The listing builds one solid part. Answer for the finished solid, in the listing's coordinates (mm). Face numbers are marked on the shaded views. A direction names the side the tool comes from. Round coordinates to 2 decimals unless told otherwise and drop trailing zeros. Write each loop counter-clockwise with the first axis right and the second up, starting at its lowest first coordinate (ties: lowest second). Pieces come first, ordered by that corner, then holes.
Item 1: Each of these flat-tipped pins is pushed along its axis until it touches: pin 1 (2 mm diameter, centred on x = -5, y = 16.5, fed in from -Z); pin 2 (0.8 mm diameter, centred on y = 13, z = 1, fed in from -X); pin 3 (2 mm diameter, centred on y = 21, z = 0, fed in from +X) (3 decimals); pin 4 (3.5 mm diameter, centred on x = 0, y = 44, fed in from +Z). Where does it stop, or does it pass through?
Item 2: Find section A-A on y = 16. Give the vertices of the cut face in (x, z) (3 decimals), then the cut area to 4 significant figures.
Item 3: For a pull along Y with two mould halves and no side action, classify the marked faces 1, 2, 3 and 4 as +Y half, -Y half, draft (parallel to the pull), parting line (faces both ways), or undercut.
Item 4: Find section B-B on y = 25. Give the vertices of the cut face in (x, z).
Item 5: Find the intervals of material crossed by probe 1 along X at (y, z) = (36, 0.75); probe 2 along X at (y, z) = (20, -1.25) (3 decimals); probe 3 along Z at (x, y) = (1, 45), in increasing order.
Item 6: A tool of negligible diameter and unlimited length cuts with its end or side. For the marked faces 5, 6 and 7, from which of +Z, -Z, +X, -X, +Y, -Y can it reach the whole face along a straight path? Write none if from no direction.
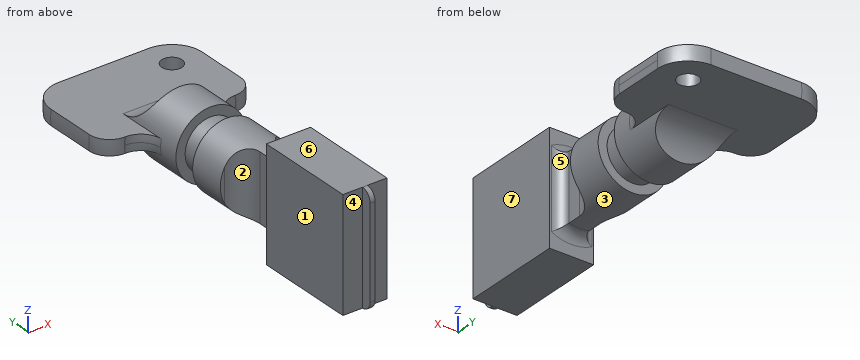
```python
from build123d import *

# Parameters (mm, degrees)
BOSS_EXTRUDE1_DEPTH      = 10
FILLET2_R                = 2
FILLET3_R                = 3
CUT_EXTRUDE1_DEPTH       = 49.473897211
CUT_EXTRUDE1_DEPTH_BACK  = 49.473897211
SKETCH3_R                = 1
CUT_EXTRUDE2_DEPTH       = 49.473897211
CUT_EXTRUDE2_DEPTH_BACK  = 49.473897211
SKETCH4_W                = 5.555619824
SKETCH4_H                = 11.886700215
SKETCH4_W_2              = 4.837610552
SKETCH4_H_2              = 13.886700215
FILLET4_R                = 2
BOSS_EXTRUDE2_DEPTH      = 5.5
BOSS_EXTRUDE2_DEPTH_BACK = 5.5
SKETCH7_W                = 4.35
SKETCH7_H                = 10
FILLET5_R                = 1
SKETCH8_W                = 0.486068648
SKETCH8_H                = 11
BOSS_EXTRUDE3_DEPTH      = 1
FILLET6_R                = 1


with BuildPart() as part:
    # Sketch1 → Revolve1 (revolve)
    with BuildSketch(Plane.XY):
        Polygon((-3.448914015, 37.765821371), (-3.448914015, 33.765821371), (-2.534753992, 33.765821371), (-2.534753992, 31.624967984), (-3.41766068, 31.624967984), (-3.41766068, 23), (0, 23), (0, 37.765821371), align=None)
    revolve(axis=Axis((0, 37.765821371, 0), (0, -1, 0)))

    # Sketch2 → Boss-Extrude1 (add)
    with BuildSketch(Plane(origin=(0, 37.765821371, 0), x_dir=(1, 0, 0), z_dir=(0, 1, 0))):
        with BuildLine():
            Line((3.366379046, 0.75), (-3.366379046, 0.75))
            ThreePointArc((-3.366379046, 0.75), (-3.448914015, 0), (-3.366379046, -0.75))
            Line((-3.366379046, -0.75), (3.366379046, -0.75))
            ThreePointArc((3.366379046, -0.75), (3.428218178, -0.37726384), (3.448914015, 0))
            ThreePointArc((3.448914015, 0), (3.428218178, 0.37726384), (3.366379046, 0.75))
        make_face()
        with BuildLine():
            Line((-3.366379046, 0.75), (-7.462405778, 0.75))
            ThreePointArc((-7.462405778, 0.75), (-7.5, 0), (-7.462405778, -0.75))
            Line((-7.462405778, -0.75), (-3.366379046, -0.75))
            ThreePointArc((-3.366379046, -0.75), (-3.448914015, 0), (-3.366379046, 0.75))
        make_face()
        with BuildLine():
            ThreePointArc((7.5, 0), (7.490595548, 0.375470813), (7.462405778, 0.75))
            Line((7.462405778, 0.75), (3.366379046, 0.75))
            ThreePointArc((3.366379046, 0.75), (3.428218178, 0.37726384), (3.448914015, 0))
            ThreePointArc((3.448914015, 0), (3.428218178, -0.37726384), (3.366379046, -0.75))
            Line((3.366379046, -0.75), (7.462405778, -0.75))
            ThreePointArc((7.462405778, -0.75), (7.490595548, -0.375470813), (7.5, 0))
        make_face()
    extrude(amount=BOSS_EXTRUDE1_DEPTH)

    # Fillet2
    # the kernel refuses this fillet: 2 mm, written as the material it adds along each edge
    with BuildSketch(Plane(origin=(0, 37.765821371, 0), x_dir=(-0.09803421101524086, 0, -0.9951830452085783), z_dir=(-0.9951830452085783, 0, 0.09803421101524086))) as fillet2_piece_1_section:
        with BuildLine():
            CenterArc((3.448914015 + FILLET2_R, FILLET2_R), FILLET2_R, 180, 90)
            Line((3.448914015 + FILLET2_R, 0), (3.448914015, 0))
            Line((3.448914015, 0), (3.448914015, FILLET2_R))
        make_face()
    fillet2_piece_1 = revolve(axis=Axis((0, 37.765821371, 0), (0, -1, 0)), revolution_arc=191.251965623, mode=Mode.PRIVATE)
    fillet2_piece_1 = split(fillet2_piece_1, bisect_by=Plane(origin=(3.870689991, 37.318827735, -0.75), z_dir=(0, 0, 1)), keep=Keep.TOP, mode=Mode.PRIVATE)
    fillet2_piece_1 = split(fillet2_piece_1, bisect_by=Plane(origin=(3.870689991, 37.318827735, 0.75), z_dir=(0, 0, -1)), keep=Keep.TOP, mode=Mode.PRIVATE)
    add(fillet2_piece_1)
    with BuildSketch(Plane(origin=(0, 37.765821371, 0), x_dir=(0.09800035789508027, 0, 0.9951863794548418), z_dir=(0.9951863794548418, 0, -0.09800035789508027))) as fillet2_piece_2_section:
        with BuildLine():
            CenterArc((3.448914015 + FILLET2_R, FILLET2_R), FILLET2_R, 180, 90)
            Line((3.448914015 + FILLET2_R, 0), (3.448914015, 0))
            Line((3.448914015, 0), (3.448914015, FILLET2_R))
        make_face()
    fillet2_piece_2 = revolve(axis=Axis((0, 37.765821371, 0), (0, -1, 0)), revolution_arc=95.624033786, mode=Mode.PRIVATE)
    fillet2_piece_2 = split(fillet2_piece_2, bisect_by=Plane(origin=(-3.870690025, 37.318827894, 0.75), z_dir=(0, 0, -1)), keep=Keep.TOP, mode=Mode.PRIVATE)
    add(fillet2_piece_2)
    with BuildSketch(Plane(origin=(0, 37.765821371, 0), x_dir=(-1, 0, 0), z_dir=(0, 0, 1))) as fillet2_piece_3_section:
        with BuildLine():
            CenterArc((3.448914015 + FILLET2_R, FILLET2_R), FILLET2_R, 180, 90)
            Line((3.448914015 + FILLET2_R, 0), (3.448914015, 0))
            Line((3.448914015, 0), (3.448914015, FILLET2_R))
        make_face()
    fillet2_piece_3 = revolve(axis=Axis((0, 37.765821371, 0), (0, -1, 0)), revolution_arc=95.624033786, mode=Mode.PRIVATE)
    fillet2_piece_3 = split(fillet2_piece_3, bisect_by=Plane(origin=(-3.870689874, 37.318828004, -0.75), z_dir=(0, 0, 1)), keep=Keep.TOP, mode=Mode.PRIVATE)
    add(fillet2_piece_3)
    # the kernel refuses this fillet: 2 mm, written as the material it takes off along each edge
    with BuildSketch(Plane(origin=(0, 37.765821371, 0), x_dir=(-0.7201079494948177, 0, -0.6938620475817721), z_dir=(0.6938620475817721, 0, -0.7201079494948177))) as fillet2_2_piece_1:
        with BuildLine():
            CenterArc((7.5 - FILLET2_R, FILLET2_R), FILLET2_R, 270, 90)
            Line((7.5, FILLET2_R), (7.5, 0))
            Line((7.5, 0), (7.5 - FILLET2_R, 0))
        make_face()
    revolve(axis=Axis((0, 37.765821371, 0), (0, 1, 0)), revolution_arc=87.873212667, mode=Mode.SUBTRACT)
    with BuildSketch(Plane(origin=(0, 37.765821371, 0), x_dir=(0.7201079494948216, 0, 0.6938620475817678), z_dir=(-0.6938620475817678, 0, 0.7201079494948216))) as fillet2_2_piece_2:
        with BuildLine():
            CenterArc((7.5 - FILLET2_R, FILLET2_R), FILLET2_R, 270, 90)
            Line((7.5 - FILLET2_R, 0), (7.5, 0))
            Line((7.5, 0), (7.5, FILLET2_R))
        make_face()
    revolve(axis=Axis((0, 37.765821371, 0), (0, 1, 0)), revolution_arc=87.873212667, mode=Mode.SUBTRACT)

    # Fillet3
    # the kernel refuses this fillet: 3 mm, written as the material it adds along each edge
    with BuildSketch(Plane(origin=(10.866379046, 37.765821371, -0.75), x_dir=(0, 1, 0), z_dir=(-1, 0, 0))) as fillet3_piece_1_section:
        with BuildLine():
            CenterArc((FILLET3_R, FILLET3_R), FILLET3_R, 180, 90)
            Line((0, FILLET3_R), (0, 0))
            Line((0, 0), (FILLET3_R, 0))
        make_face()
    fillet3_piece_1 = extrude(amount=21.732758092, mode=Mode.PRIVATE)
    fillet3_piece_1 = fillet3_piece_1 & Plane(origin=(0, 38.470226203, 0), x_dir=(-1, 0, 0), z_dir=(0, -1, 0)) * Cylinder(3.448914015, 56, mode=Mode.PRIVATE)
    add(fillet3_piece_1)
    with BuildSketch(Plane(origin=(10.866379046, 37.765821371, 0.75), x_dir=(0, 1, 0), z_dir=(-1, 0, 0))) as fillet3_piece_2_section:
        with BuildLine():
            CenterArc((FILLET3_R, -FILLET3_R), FILLET3_R, 90, 90)
            Line((0, -FILLET3_R), (0, 0))
            Line((0, 0), (FILLET3_R, 0))
        make_face()
    fillet3_piece_2 = extrude(amount=21.732758092, mode=Mode.PRIVATE)
    fillet3_piece_2 = fillet3_piece_2 & Plane(origin=(0, 38.470226203, 0), x_dir=(-1, 0, 0), z_dir=(0, -1, 0)) * Cylinder(3.448914015, 56, mode=Mode.PRIVATE)
    add(fillet3_piece_2)
    # the kernel refuses this fillet: 3 mm, written as the material it takes off along each edge
    with BuildSketch(Plane(origin=(0, 47.765821371, 0), x_dir=(-0.4534410859899706, 0, -0.8912862511764871), z_dir=(0.8912862511764871, 0, -0.4534410859899706))) as fillet3_2_piece_1:
        with BuildLine():
            CenterArc((7.5 - FILLET3_R, -FILLET3_R), FILLET3_R, 0, 90)
            Line((7.5 - FILLET3_R, 0), (7.5, 0))
            Line((7.5, 0), (7.5, -FILLET3_R))
        make_face()
    revolve(axis=Axis((0, 47.765821371, 0), (0, 1, 0)), revolution_arc=126.070648523, mode=Mode.SUBTRACT)
    with BuildSketch(Plane(origin=(0, 47.765821371, 0), x_dir=(0.4534410859901425, 0, -0.8912862511763997), z_dir=(-0.8912862511763997, 0, -0.4534410859901425))) as fillet3_2_piece_2:
        with BuildLine():
            CenterArc((7.5 - FILLET3_R, FILLET3_R), FILLET3_R, 270, 90)
            Line((7.5, FILLET3_R), (7.5, 0))
            Line((7.5, 0), (7.5 - FILLET3_R, 0))
        make_face()
    revolve(axis=Axis((0, 47.765821371, 0), (0, -1, 0)), revolution_arc=126.070648523, mode=Mode.SUBTRACT)

    # Sketch3 → Cut-Extrude1 (cut, two sides: drawn at the far end of the back side and taken through both)
    with BuildSketch(Plane.XY.offset(-CUT_EXTRUDE1_DEPTH_BACK)):
        with Locations((4.462405778, 44.765821371)):
            Circle(SKETCH3_R)
    extrude(amount=CUT_EXTRUDE1_DEPTH + CUT_EXTRUDE1_DEPTH_BACK, mode=Mode.SUBTRACT)

    # Sketch4 → Cut-Extrude2 (cut, two sides: drawn at the far end of the back side and taken through both)
    with BuildSketch(Plane.XY.offset(-CUT_EXTRUDE2_DEPTH_BACK)):
        with Locations((-3.777809912, 22.056649893)):
            Rectangle(SKETCH4_W, SKETCH4_H)
        with Locations((3.418805276, 21.056649893)):
            Rectangle(SKETCH4_W_2, SKETCH4_H_2)
    extrude(amount=CUT_EXTRUDE2_DEPTH + CUT_EXTRUDE2_DEPTH_BACK, mode=Mode.SUBTRACT)

    # Fillet4
    fillet4_edges = [part.edges().sort_by_distance(p)[0] for p in [
        (-1, 28, 0),
        (1, 28, 0),
    ]]
    fillet(fillet4_edges, radius=FILLET4_R)

    # Sketch7 → Boss-Extrude2 (add, two sides: drawn at the far end of the back side and taken through both)
    with BuildSketch(Plane.XY.offset(-BOSS_EXTRUDE2_DEPTH_BACK)):
        with Locations((0, 18.624967984)):
            Rectangle(SKETCH7_W, SKETCH7_H)
    extrude(amount=BOSS_EXTRUDE2_DEPTH + BOSS_EXTRUDE2_DEPTH_BACK)

    # Fillet5
    fillet5_edges = [part.edges().sort_by_distance(p)[0] for p in [
        (1, 23.624967984, 0),
        (0, 23.624967984, -3.41766068),
        (0, 23.624967984, 3.41766068),
        (-1, 23.624967984, 0),
    ]]
    fillet(fillet5_edges, radius=FILLET5_R)

    # Sketch8 → Boss-Extrude3 (add)
    with BuildSketch(Plane.XZ.offset(-13.624967984)):
        Rectangle(SKETCH8_W, SKETCH8_H)
    extrude(amount=BOSS_EXTRUDE3_DEPTH)

    # Fillet6
    fillet6_edges = [part.edges().sort_by_distance(p)[0] for p in [
        (0, 12.624967984, -5.5),
        (0, 12.624967984, 5.5),
    ]]
    fillet(fillet6_edges, radius=FILLET6_R)


solid = part.part
```
Check values:
1. pin 1: passes through
1. pin 2: stops at x = -0.24
1. pin 3: stops at x = 2.175
1. pin 4: stops at z = 0.75
2. outline: (-2.175, -5.5) - (2.175, -5.5) - (2.175, 5.5) - (-2.175, 5.5) - close
2. area: 47.85 mm2
3. face 1: draft
3. face 2: undercut
3. face 3: undercut
3. face 4: -Y half
4. outline: (-1, -3.27) arc R3.42 ccw to (1, -3.27) - (1, 3.27) arc R3.42 ccw to (-1, 3.27) - close
5. probe 1: x = -3.37 to 3.37
5. probe 2: x = -2.175 to 2.175
5. probe 3: z = -0.75 to 0.75
6. face 5: +Z, -Z, +X
6. face 6: +Z, +X, -X, +Y, -Y
6. face 7: +Z, -Z, +X, -Y
